```python
from build123d import *

# Parameters (mm, degrees)
INLAY_PROFILE_DEPTH = 1.524


with BuildPart() as part:
    # Sketch1 → Inlay Profile (new body)
    with BuildSketch(Plane.XY.offset(317.1825)):
        with BuildLine():
            Line((18.025571565, -0.367457164), (4.664168889, 12.994014038))
            add(Edge.make_bspline(
                [(4.664168889, 12.994014038), (4.356818389, 13.301283177), (4.023428442, 13.576107861), (3.303188568, 14.059147528), (2.921540553, 14.263277993), (2.327729087, 14.509301237), (2.125703276, 14.581569814), (1.713361811, 14.706360576), (1.502025353, 14.759048678), (0.864474651, 14.884719032), (0.434602166, 14.926131934), (0, 14.926131934)],
                knots=[0, 0, 0, 0, 0.25, 0.25, 0.5, 0.5, 0.625, 0.625, 0.75, 0.75, 1, 1, 1, 1], degree=3))
            add(Edge.make_bspline(
                [(0, 14.926131934), (-0.434565559, 14.926131934), (-0.864598328, 14.884737713), (-1.715362235, 14.717005142), (-2.129530035, 14.591455059), (-2.723303198, 14.345481802), (-2.91723014, 14.253710711), (-3.296979358, 14.050339945), (-3.483640779, 13.938135256), (-4.023200182, 13.576118838), (-4.356357054, 13.301389905), (-4.663566812, 12.994033668)],
                knots=[0, 0, 0, 0, 0.25, 0.25, 0.5, 0.5, 0.625, 0.625, 0.75, 0.75, 1, 1, 1, 1], degree=3))
            Line((-4.663566812, 12.994033668), (-18.025649465, -0.367432276))
            add(Edge.make_bspline(
                [(-18.025649465, -0.367432276), (-18.333467155, -0.67533686), (-18.606471867, -1.007956137), (-18.964627192, -1.543341075), (-19.075411795, -1.727908456), (-19.279353822, -2.109557241), (-19.372638179, -2.307251324), (-19.619790253, -2.906272044), (-19.743635222, -3.317359375), (-19.911015551, -4.162573597), (-19.953704554, -4.599216881), (-19.953952622, -5.459245308), (-19.912854372, -5.886970886), (-19.787519071, -6.525023338), (-19.734956892, -6.736784446), (-19.61063072, -7.149788503), (-19.538661355, -7.352219952), (-19.293631903, -7.947426043), (-19.090333968, -8.330215541), (-18.607972779, -9.052961748), (-18.333143835, -9.387372973), (-18.025264594, -9.695301528)],
                knots=[0, 0, 0, 0, 0.125, 0.125, 0.1875, 0.1875, 0.25, 0.25, 0.375, 0.375, 0.5, 0.5, 0.625, 0.625, 0.6875, 0.6875, 0.75, 0.75, 0.875, 0.875, 1, 1, 1, 1], degree=3))
            Line((-18.025264594, -9.695301528), (-4.663524615, -23.056904469))
            add(Edge.make_bspline(
                [(-4.663524615, -23.056904469), (-4.356310087, -23.364249214), (-4.023007479, -23.63909939), (-3.302884908, -24.122140042), (-2.921265042, -24.326244773), (-2.327500967, -24.572212863), (-2.12549016, -24.644461146), (-1.713179231, -24.769212535), (-1.501858849, -24.82188113), (-0.864378385, -24.94749901), (-0.434553406, -24.988892008), (0, -24.988892008)],
                knots=[0, 0, 0, 0, 0.25, 0.25, 0.5, 0.5, 0.625, 0.625, 0.75, 0.75, 1, 1, 1, 1], degree=3))
            add(Edge.make_bspline(
                [(0, -24.988892008), (0.434598725, -24.988892008), (0.864662427, -24.947480808), (1.715485434, -24.779696058), (2.129672534, -24.65411367), (2.723485659, -24.408109873), (2.917427142, -24.316331785), (3.29721076, -24.112960431), (3.48389071, -24.000763389), (4.02353835, -23.638788642), (4.356791056, -23.364119061), (4.664144191, -23.05686733)],
                knots=[0, 0, 0, 0, 0.25, 0.25, 0.5, 0.5, 0.625, 0.625, 0.75, 0.75, 1, 1, 1, 1], degree=3))
            Line((4.664144191, -23.05686733), (18.025583545, -9.695290931))
            add(Edge.make_bspline(
                [(18.025583545, -9.695290931), (18.333482821, -9.387431146), (18.606580042, -9.054852177), (18.964876906, -8.519511604), (19.07570919, -8.334956341), (19.279745495, -7.953324821), (19.373075727, -7.75563737), (19.620355994, -7.156630228), (19.744276575, -6.745539993), (19.911775941, -5.900292811), (19.954506627, -5.463624258), (19.954794901, -4.60354651), (19.913696633, -4.175791487), (19.788326474, -3.537687683), (19.735750086, -3.325922766), (19.611387505, -2.912908888), (19.539395757, -2.710472584), (19.294286623, -2.115252142), (19.090902314, -1.732430795), (18.608415217, -1.009737255), (18.333518116, -0.67535632), (18.025571565, -0.367457164)],
                knots=[0, 0, 0, 0, 0.125, 0.125, 0.1875, 0.1875, 0.25, 0.25, 0.375, 0.375, 0.5, 0.5, 0.625, 0.625, 0.6875, 0.6875, 0.75, 0.75, 0.875, 0.875, 1, 1, 1, 1], degree=3))
        make_face()
        with BuildLine():
            Line((2.764163115, -18.666741649), (13.243958907, -8.185849192))
            add(Edge.make_bspline(
                [(13.243958907, -8.185849192), (13.608833555, -7.821914197), (13.899676587, -7.388141491), (14.191534414, -6.683923004), (14.266383768, -6.43680018), (14.365551211, -5.933629733), (14.390147378, -5.678984441), (14.390147378, -5.42132701)],
                knots=[0, 0, 0, 0, 0.5, 0.5, 0.75, 0.75, 1, 1, 1, 1], degree=3))
            add(Edge.make_bspline(
                [(14.390147378, -5.42132701), (14.390147378, -4.906143502), (14.288977165, -4.393966558), (13.997180838, -3.689977029), (13.875278396, -3.462430015), (13.589364349, -3.036852796), (13.426546706, -2.839620383), (13.244193351, -2.657689678)],
                knots=[0, 0, 0, 0, 0.5, 0.5, 0.75, 0.75, 1, 1, 1, 1], degree=3))
            add(Edge.make_bspline(
                [(13.244193351, -2.657689678), (11.84504508, -1.258501699), (10.445900405, 0.14068981), (9.046761495, 1.539887083), (7.752789848, 2.833912707), (6.458822874, 4.127943003), (5.164865581, 5.421982981), (3.870908288, 6.716022958), (2.576957547, 8.010069489), (1.283039711, 9.304148919)],
                knots=[0, 0, 0, 0, 0.005936167, 0.005936167, 0.005936167, 0.011426139, 0.011426139, 0.011426139, 0.01691611, 0.01691611, 0.01691611, 0.01691611], degree=3))
            add(Edge.make_bspline(
                [(1.283039711, 9.304148919), (1.208451812, 9.37880166), (1.128215528, 9.445680851), (0.955177572, 9.562146218), (0.861064542, 9.612149298), (0.666716276, 9.688920917), (0.566349911, 9.716183545), (0.359200688, 9.74835085), (0.253130484, 9.752841938), (-0.059388996, 9.733662582), (-0.265779648, 9.677263143), (-0.64537994, 9.499967758), (-0.819554471, 9.379722795), (-1.123868056, 9.091145072), (-1.252509124, 8.924477208), (-1.398287945, 8.647032516), (-1.439236675, 8.548793299), (-1.500120392, 8.349062122), (-1.52065849, 8.24669022), (-1.538945102, 8.036179126), (-1.536277907, 7.931558062), (-1.507085794, 7.725573364), (-1.479946725, 7.622528868), (-1.364975159, 7.329677155), (-1.243195343, 7.153930867), (-1.093632727, 7.004481006)],
                knots=[0, 0, 0, 0, 0.0625, 0.0625, 0.125, 0.125, 0.1875, 0.1875, 0.25, 0.25, 0.375, 0.375, 0.5, 0.5, 0.625, 0.625, 0.6875, 0.6875, 0.75, 0.75, 0.8125, 0.8125, 0.875, 0.875, 1, 1, 1, 1], degree=3))
            add(Edge.make_bspline(
                [(-1.093632727, 7.004481006), (0.253348837, 5.656986284), (1.600507848, 4.309668958), (2.947696525, 2.962381313), (4.187919425, 1.722067304), (5.428183671, 0.481794636), (6.668468389, -0.758457558), (7.908753108, -1.998709755), (9.149059402, -3.238940377), (10.389379137, -4.479157555)],
                knots=[0, 0, 0, 0, 0.005715847, 0.005715847, 0.005715847, 0.010977861, 0.010977861, 0.010977861, 0.016239874, 0.016239874, 0.016239874, 0.016239874], degree=3))
            ThreePointArc((10.389379137, -4.479157555), (10.77999123, -5.422091507), (10.389424288, -6.36504416))
            Line((10.389424288, -6.36504416), (0.943369001, -15.811222968))
            ThreePointArc((0.943369001, -15.811222968), (0.000426035, -16.20180224), (-0.942511126, -15.811208956))
            Line((-0.942511126, -15.811208956), (-4.907243278, -11.846307125))
            ThreePointArc((-4.907243278, -11.846307125), (-5.297796208, -10.903342622), (-4.907161552, -9.960411971))
            add(Edge.make_bspline(
                [(-4.907161552, -9.960411971), (-4.017282762, -9.070649343), (-3.127409839, -8.180880848), (-2.237548499, -7.291100768), (-1.534518938, -6.588135406), (-0.831496023, -5.885163397), (-0.128489581, -5.182174915), (0.574516863, -4.47918643), (1.277525983, -3.776200612), (1.980431653, -3.073111364)],
                knots=[0, 0, 0, 0, 0.00377519, 0.00377519, 0.00377519, 0.006757755, 0.006757755, 0.006757755, 0.009740321, 0.009740321, 0.009740321, 0.009740321], degree=3))
            add(Edge.make_bspline(
                [(1.980431653, -3.073111364), (2.140804197, -2.912661242), (2.282926924, -2.73900393), (2.456044926, -2.449522576), (2.507357822, -2.3470096), (2.589643367, -2.13613991), (2.620897599, -2.027784662), (2.67933703, -1.692286826), (2.668256404, -1.461430231), (2.56455456, -1.136554805), (2.516796459, -1.034532881), (2.395068593, -0.842948012), (2.321446097, -0.754709164), (2.156381432, -0.600330836), (2.062934312, -0.532455362), (1.865547855, -0.421945587), (1.760257054, -0.378198331), (1.541383287, -0.314868209), (1.430053085, -0.29575808), (1.203867431, -0.280914383), (1.089027609, -0.285532444), (0.753475716, -0.332291796), (0.535040575, -0.408379414), (0.137984232, -0.6245314), (-0.043673421, -0.765401767), (-0.204860953, -0.926528537)],
                knots=[0, 0, 0, 0, 0.125, 0.125, 0.1875, 0.1875, 0.25, 0.25, 0.375, 0.375, 0.4375, 0.4375, 0.5, 0.5, 0.5625, 0.5625, 0.625, 0.625, 0.6875, 0.6875, 0.75, 0.75, 0.875, 0.875, 1, 1, 1, 1], degree=3))
            add(Edge.make_bspline(
                [(-0.204860953, -0.926528537), (-0.641101053, -1.362793519), (-1.077372199, -1.799027457), (-1.513647836, -2.235256899), (-2.440333949, -3.161844889), (-3.367052449, -4.088400488), (-4.293778224, -5.014948809), (-5.220504, -5.941497132), (-6.147239872, -6.868035357), (-7.073980722, -7.794568602)],
                knots=[0, 0, 0, 0, 0.001850863, 0.001850863, 0.001850863, 0.005782251, 0.005782251, 0.005782251, 0.009713639, 0.009713639, 0.009713639, 0.009713639], degree=3))
            ThreePointArc((-7.073980722, -7.794568602), (-8.017129764, -8.185036049), (-8.960086733, -7.794104987))
            Line((-8.960086733, -7.794104987), (-10.389194361, -6.363911994))
            ThreePointArc((-10.389194361, -6.363911994), (-10.779409558, -5.420973836), (-10.388672202, -4.478251932))
            add(Edge.make_bspline(
                [(-10.388672202, -4.478251932), (-9.620363184, -3.710210592), (-8.852080067, -2.942143342), (-8.083834335, -2.174038699), (-7.262017343, -1.352372632), (-6.440241976, -0.530664926), (-5.618537443, 0.291113605), (-4.796832885, 1.11289216), (-3.975193451, 1.934735858), (-3.153705857, 2.7567313)],
                knots=[0, 0, 0, 0, 0.003259091, 0.003259091, 0.003259091, 0.006745445, 0.006745445, 0.006745445, 0.0102318, 0.0102318, 0.0102318, 0.0102318], degree=3))
            add(Edge.make_bspline(
                [(-3.153705857, 2.7567313), (-3.073275327, 2.837120342), (-3.001018869, 2.923298121), (-2.874183174, 3.108172399), (-2.819145258, 3.207947086), (-2.731427392, 3.416662057), (-2.699146348, 3.523975917), (-2.657489826, 3.744452491), (-2.648280145, 3.858971027), (-2.662206408, 4.422495916), (-2.86542486, 4.865755486), (-3.274203407, 5.251671073), (-3.365231629, 5.321829449), (-3.556910695, 5.439619692), (-3.657999963, 5.488005812), (-3.978069809, 5.599529591), (-4.20753438, 5.624830423), (-4.545641744, 5.586274821), (-4.655458789, 5.56134804), (-4.869936225, 5.489914826), (-4.974382972, 5.443189754), (-5.269396668, 5.280222942), (-5.447707363, 5.138839656), (-5.608265037, 4.978375432)],
                knots=[0, 0, 0, 0, 0.0625, 0.0625, 0.125, 0.125, 0.1875, 0.1875, 0.25, 0.25, 0.5, 0.5, 0.5625, 0.5625, 0.625, 0.625, 0.75, 0.75, 0.8125, 0.8125, 0.875, 0.875, 1, 1, 1, 1], degree=3))
            add(Edge.make_bspline(
                [(-5.608265037, 4.978375432), (-6.419093367, 4.167567138), (-7.229912955, 3.356750104), (-8.04072861, 2.545929136), (-8.907975502, 1.67867656), (-9.775217571, 0.811419162), (-10.642456843, -0.055841034), (-11.509696114, -0.92310123), (-12.376932511, -1.7903643), (-13.244166976, -2.657629303)],
                knots=[0, 0, 0, 0, 0.003440011, 0.003440011, 0.003440011, 0.00711944, 0.00711944, 0.00711944, 0.010798869, 0.010798869, 0.010798869, 0.010798869], degree=3))
            add(Edge.make_bspline(
                [(-13.244166976, -2.657629303), (-13.608600195, -3.021827623), (-13.899427442, -3.455428378), (-14.191343401, -4.159425647), (-14.266223067, -4.406472325), (-14.365420486, -4.909539259), (-14.390010332, -5.164133807), (-14.390010332, -5.421738148)],
                knots=[0, 0, 0, 0, 0.5, 0.5, 0.75, 0.75, 1, 1, 1, 1], degree=3))
            add(Edge.make_bspline(
                [(-14.390010332, -5.421738148), (-14.390010332, -5.936941134), (-14.288825943, -6.449133342), (-13.997063, -7.153166102), (-13.875183954, -7.38072782), (-13.589321969, -7.806370664), (-13.426536962, -8.003645163), (-13.244218716, -8.185623942)],
                knots=[0, 0, 0, 0, 0.5, 0.5, 0.75, 0.75, 1, 1, 1, 1], degree=3))
            Line((-13.244218716, -8.185623942), (-2.764136748, -18.664986339))
            add(Edge.make_bspline(
                [(-2.764136748, -18.664986339), (-2.400035433, -19.029574977), (-1.966546507, -19.320649385), (-1.262547507, -19.612746574), (-1.015462867, -19.68766307), (-0.512378601, -19.786880045), (-0.257767564, -19.811465257), (-0.000142467, -19.811474386)],
                knots=[0, 0, 0, 0, 0.5, 0.5, 0.75, 0.75, 1, 1, 1, 1], degree=3))
            add(Edge.make_bspline(
                [(-0.000142467, -19.811474386), (0.515090813, -19.812034072), (1.027360033, -19.71098374), (1.731500271, -19.419371754), (1.959103087, -19.297532052), (2.384821027, -19.011767969), (2.582144098, -18.849033097), (2.764163115, -18.666741649)],
                knots=[0, 0, 0, 0, 0.5, 0.5, 0.75, 0.75, 1, 1, 1, 1], degree=3))
        make_face(mode=Mode.SUBTRACT)
    extrude(amount=-INLAY_PROFILE_DEPTH)


solid = part.part
```
Work out the finished part from the listing and answer in its coordinate system (mm). A direction names the side the tool comes from. Give positions to 0.01 mm unless a question says otherwise; leave off trailing zeros. Write each loop counter-clockwise with the first axis right and the second up, starting at its lowest first coordinate (ties: lowest second). Pieces come first, ordered by that corner, then holes. Notation, with made-up numbers: (50.25, -3) -> (69.25, -3) arc R27 cw to (69.25, 21) -> close; hole circle Ø9 at (2.25, -27.5). An arc over 180 degrees is marked (long way). Write each question's results on one line, items separated by ' | '.
1. Find section D-D on y = 11. Determine the outline of the cut face in (x, z).
Data:
outline: (-6.66, 315.66) -> (6.66, 315.66) -> (6.66, 317.18) -> (-6.66, 317.18) -> close
2. Straight lines are drawn through the part: L1, parallel to Y at x = 1.5, z = 316; L2, parallel to X at y = -16, z = 316.4; L3, parallel to X at y = -13.5, z = 316.9. For each, find the intervals that lie inside material, in ascending order.
Data:
L1: -24.82 to -19.52, -15.25 to -3.55, -0.31 to 4.41, 9.09 to 14.76 | L2: -11.72 to -5.43, -0.7 to 0.71, 5.43 to 11.72 | L3: -14.22 to -7.93, -3.25 to 3.25, 7.93 to 14.22
3. Find section A-A on x = 7.5. Give the number of separate pieces and of enclosed holes in the cut face, and give its area (3 significant figures).
Data:
separate pieces: 3 | enclosed holes: 0 | area: 32.0 mm^2
4. A tool of negligible diameter and unlimited length cuts with its end or side. For faces 1 (the flat face through (11.25, -16.47, 316.43)), 2 (the flat face through (-2.897, -13.857, 316.431)), from which of +Z, -Z, +X, -X, +Y, -Y can it reach the whole face along a straight path? Write none if from no direction.
Data:
face 1: +Z, -Z, +X, -Y | face 2: +Z, -Z
5. Determine the mould class of faces 3 (the flat face through (-11.44, -16.28, 316.43)), 4 (the flat face through (11.44, 6.22, 316.43)), 5 (the cylindrical face through (10.78, -5.41, 316.43)) for opening direction Y: +Y half, -Y half, draft (parallel to the pull), parting line (faces both ways), or undercut.
Data:
face 3: -Y half | face 4: +Y half | face 5: undercut
6. This flat-tipped pin is pushed along its axis until it touches: pin 1 Ø3 at (x, y) = (-9.5, -20.5) entering from +Z (3 decimals). Where does it stop, or does it pass through?
Data:
pin 1: through
